Read the model definition and answer for the solid it produces. Units are mm, in the model's axes. A direction names the side the tool comes from. Coordinates: 2 decimals unless noted, no trailing zeros. Write each loop counter-clockwise with the first axis right and the second up, starting at its lowest first coordinate (ties: lowest second). Pieces come first, ordered by that corner, then holes.
Item 1: Determine the mould class of faces 1 (the face through (-44.369, -7.042, -3.327)), 2 (the face through (12.912, -4.93, -32.451)), 3 (the face through (-25, 0, -9)) for opening direction Z: released by +Z, released by -Z, zero draft, split by the parting line, or undercut.
Item 2: Section C-C (x = 16.5) is taken. Give the vertices of the cut face in (y, z), then the cut area to 3 significant figures.
Item 3: Section B-B (z = -18) is taken. Give the vertices of the cut face in (x, y), then the cut area to 3 significant figures.
Item 4: A tool of negligible diameter and unlimited length cuts with its end or side. For faces 4 (the face through (-48, -5, 16)), 5 (the face through (-45.7, -7, -1)), 6 (the face through (-73, -5, -15)), from which of +Z, -Z, +X, -X, +Y, -Y can it reach the whole face along a straight path? Write none if from no direction.
Item 5: Section A-A (y = -2.75) is taken. State how many separate pieces and enclosed holes the cut face has, then the cut area to 3 significant figures.
Item 6: Each of these flat-tipped pins is pushed along its axis until it touches: P1, Ø3, axis at y = -6.5, z = -40, coming from the +X side; P2, Ø8, axis at x = 0, z = 0, coming from the -Y side; P3, Ø2.5, axis at x = -44, z = -1.5, coming from the -Y side; P4, Ø2.5, axis at y = -6.5, z = -1.5, coming from the +X side. Where does it stop, or does it pass through?
Item 7: Section D-D (z = 25) is taken. Give the vertices of the cut face in (x, y).
Item 8: Straight lines are drawn through the part: probe 1 along Z at (x, y) = (-37, -1.5); probe 2 along X at (y, z) = (-0.75, -29.5); probe 3 along Z at (x, y) = (-46, -0.25). For each, find the intervals that lie inside material, in ascending order.
from build123d import *

# Parameters (mm, degrees)
SKETCH_R        = 2.425
SKETCH_R_2      = 1.925
PAD_DEPTH       = 10
POCKET_DEPTH    = 12
SKETCH002_R     = 1.925
POCKET001_DEPTH = 12
SKETCH003_R     = 1.5
POCKET002_DEPTH = 12
POCKET003_DEPTH = 6
CHAMFER_SIZE    = 2


with BuildPart() as part:
    # Sketch → Pad (new body)
    with BuildSketch(Plane.XZ):
        with BuildLine():
            ThreePointArc((12, -31.811947), (25.543993, 22.438904), (-30, 16))
            Line((-30, 16), (-67, 16))
            ThreePointArc((-67, 16), (-68.919984, 15.616672), (-70.545574, 14.525465))
            Line((-83, 2), (-70.545574, 14.525465))
            Line((-83, -54), (-83, 2))
            Line((-83, -54), (12, -54))
            Line((12, -54), (12, -31.811947))
        make_face()
        Circle(SKETCH_R, mode=Mode.SUBTRACT)
        with Locations((-67, 11)):
            Circle(SKETCH_R_2, mode=Mode.SUBTRACT)
    extrude(amount=PAD_DEPTH)

    # Sketch001 (on Face11 of Pad) → Pocket (cut)
    with BuildSketch(Plane.XZ.offset(10)):
        with BuildLine():
            ThreePointArc((-62, -4), (-73, -15), (-62, -26))
            Line((-62, -26), (-52, -26))
            ThreePointArc((-52, -26), (-41, -15), (-52, -4))
            Line((-52, -4), (-62, -4))
        make_face()
        with BuildLine():
            ThreePointArc((-77.5, 2), (-79, 0.5), (-77.5, -1))
            Line((-77.5, -1), (-67.5, -1))
            ThreePointArc((-67.5, -1), (-66, 0.5), (-67.5, 2))
            Line((-67.5, 2), (-77.5, 2))
        make_face()
        with BuildLine():
            ThreePointArc((-77.5, -29), (-79, -30.5), (-77.5, -32))
            Line((-77.5, -32), (-67.5, -32))
            ThreePointArc((-67.5, -32), (-66, -30.5), (-67.5, -29))
            Line((-67.5, -29), (-77.5, -29))
        make_face()
        with BuildLine():
            ThreePointArc((-46.5, -29), (-48, -30.5), (-46.5, -32))
            Line((-46.5, -32), (-36.5, -32))
            ThreePointArc((-36.5, -32), (-35, -30.5), (-36.5, -29))
            Line((-36.5, -29), (-46.5, -29))
        make_face()
    extrude(amount=-POCKET_DEPTH, mode=Mode.SUBTRACT)

    # Sketch002 (on Face5 of Pocket) → Pocket001 (cut)
    with BuildSketch(Plane.XZ.offset(10)):
        with Locations((-69, -49)):
            Circle(SKETCH002_R)
        with Locations((-23, -49)):
            Circle(SKETCH002_R)
        with Locations((2, -49)):
            Circle(SKETCH002_R)
    extrude(amount=-POCKET001_DEPTH, mode=Mode.SUBTRACT)

    # Sketch003 (on Face5 of Pocket001) → Pocket002 (cut)
    with BuildSketch(Plane.XZ.offset(10)):
        with Locations((-43, -1)):
            Circle(SKETCH003_R)
    extrude(amount=-POCKET002_DEPTH, mode=Mode.SUBTRACT)

    # Sketch004 (on Face5 of Pocket002) → Pocket003 (cut)
    with BuildSketch(Plane.XZ.offset(10)):
        Polygon((-43, -4.117691), (-40.3, -2.558846), (-40.3, 0.558846), (-43, 2.117691), (-45.7, 0.558846), (-45.7, -2.558846), align=None)
    extrude(amount=-POCKET003_DEPTH, mode=Mode.SUBTRACT)

    # Chamfer
    chamfer_edges = [part.edges().sort_by_distance(p)[0] for p in [
        (12, -5, -31.811947),
    ]]
    chamfer(chamfer_edges, length=CHAMFER_SIZE)


solid = part.part
Established:
1. face 1: undercut
1. face 2: released by -Z
1. face 3: zero draft
2. outline: (-10, -29.73) - (0, -29.73) - (0, 29.73) - (-10, 29.73) - close
2. area: 595 mm2
3. outline: (-83, -10) - (-72.58, -10) - (-72.58, 0) - (-83, 0) - close; (-41.42, -10) - (28.84, -10) - (28.84, 0) - (-41.42, 0) - close
3. area: 807 mm2
4. face 4: +Z, -X, +Y, -Y
4. face 5: -Y
4. face 6: +Y, -Y
5. separate pieces: 1
5. enclosed holes: 10
5. area: 7,380 mm2
6. P1: stops at x = 12
6. P2: stops at y = -10
6. P3: stops at y = -4
6. P4: stops at x = 34
7. outline: (-23.04, -10) - (23.04, -10) - (23.04, 0) - (-23.04, 0) - close
8. probe 1: z = -54 to -32, -29 to 16
8. probe 2: x = -83 to -78.62, -66.38 to -47.62, -35.38 to 16.9
8. probe 3: z = -54 to -32, -29 to -24.22, -5.78 to 16
